from build123d import *

# Parameters (mm, degrees)
SKETCH1_W           = 165.1
SKETCH1_H           = 114.3
BOSS_EXTRUDE1_DEPTH = 3
SKETCH2_W           = 100
SKETCH2_H           = 38
CUT_EXTRUDE1_DEPTH  = 4
FILLET2_R           = 10
SKETCH3_R           = 1
CUT_EXTRUDE3_DEPTH  = 4


with BuildPart() as part:
    # Sketch1 → Boss-Extrude1 (new body)
    with BuildSketch(Plane(origin=(0, 0, 0), x_dir=(1, 0, 0), z_dir=(0, 1, 0))):
        Rectangle(SKETCH1_W, SKETCH1_H)
    extrude(amount=BOSS_EXTRUDE1_DEPTH)

    # Sketch2 → Cut-Extrude1 (cut, through all)
    with BuildSketch(Plane(origin=(0, 3, 0), x_dir=(1, 0, 0), z_dir=(0, 1, 0))):
        with Locations((-32.55, -38.15)):
            Rectangle(SKETCH2_W, SKETCH2_H)
    extrude(amount=-CUT_EXTRUDE1_DEPTH, mode=Mode.SUBTRACT)

    # Fillet2
    fillet2_edges = [part.edges().sort_by_distance(p)[0] for p in [
        (-82.55, 1.5, 19.15),
        (17.45, 1.5, 57.15),
        (-82.55, 1.5, -57.15),
        (82.55, 1.5, -57.15),
        (82.55, 1.5, 57.15),
    ]]
    fillet(fillet2_edges, radius=FILLET2_R)

    # Sketch3 → Cut-Extrude3 (cut, through all)
    with BuildSketch(Plane(origin=(0, 3, 0), x_dir=(1, 0, 0), z_dir=(0, 1, 0))):
        with Locations((-52.43, 48.34)):
            Circle(SKETCH3_R)
        with Locations((-71.12, 6.35)):
            Circle(SKETCH3_R)
        with Locations((52.07, 48.34)):
            Circle(SKETCH3_R)
        with Locations((52.07, -48.26)):
            Circle(SKETCH3_R)
    extrude(amount=-CUT_EXTRUDE3_DEPTH, mode=Mode.SUBTRACT)


solid = part.part
Could you check a few things on this model? Use its own coordinates, in mm. Give positions to 0.01 mm unless a question says otherwise; leave off trailing zeros. Order: outer loops, then holes, each group sorted by start corner. A loop starts at its lowest first (then second) coordinate and runs counter-clockwise, first axis right, second up.
Item 1: I need wall thicknesses on line 1 (Z direction, x = 52.07, y = 1.2); line 2 (X direction, y = 1.45, z = -48.34); line 3 (Z direction, x = -13, y = 2.05). Which ranges of each line are inside material? Lowest first, please.
Item 2: If we section it at B-B, the plane x = -21: Write out the boundary of the cut face in (y, z).
Item 3: If we section it at A-A, the plane y = 1.5: Write out the boundary of the cut face in (x, z), plus the area to 3 significant figures.
Item 4: I'm going to push flat-ended pins straight in: pin 1 (0.9 mm diameter, centred on y = 1, z = 26.5, fed in from -X); pin 2 (0.9 mm diameter, centred on x = -32.5, y = 1, fed in from +Z); pin 3 (1.2 mm diameter, centred on x = 52.07, z = -48.34, fed in from +Y); pin 4 (10 mm diameter, centred on x = -31, z = -21.5, fed in from -Y). Where does each tip first touch, or does it pass through?
Item 5: If we section it at C-C, the plane z = 35: Write out the boundary of the cut face in (x, y), plus the area to 3 significant figures.
Values:
1. line 1: z = -57.15 to -49.34, -47.34 to 47.26, 49.26 to 57.15
1. line 2: x = -82.48 to -53.43, -51.43 to 51.07, 53.07 to 82.48
1. line 3: z = -57.15 to 19.15
2. outline: (0, -57.15) - (3, -57.15) - (3, 19.15) - (0, 19.15) - close
3. outline: (-82.55, -47.15) arc R10 ccw to (-72.55, -57.15) - (72.55, -57.15) arc R10 ccw to (82.55, -47.15) - (82.55, 47.15) arc R10 ccw to (72.55, 57.15) - (27.45, 57.15) arc R10 ccw to (17.45, 47.15) - (17.45, 19.15) - (-72.55, 19.15) arc R10 ccw to (-82.55, 9.15) - close; hole circle Ø2 at (-71.12, -6.35); hole circle Ø2 at (-52.43, -48.34); hole circle Ø2 at (52.07, -48.34); hole circle Ø2 at (52.07, 48.26)
3. area: 15,000 mm2
4. pin 1: stops at x = 17.45
4. pin 2: stops at z = 19.15
4. pin 3: passes through
4. pin 4: stops at y = 0
5. outline: (17.45, 0) - (82.55, 0) - (82.55, 3) - (17.45, 3) - close
5. area: 195 mm2
